Geometry check sheet. Reference: the model listing, model coordinates, mm. A direction names the side the tool comes from. Round coordinates to 2 decimals unless told otherwise and drop trailing zeros. Order: outer loops, then holes, each group sorted by start corner. A loop starts at its lowest first (then second) coordinate and runs counter-clockwise, first axis right, second up.
(1) Release check for a two-part mould opening along X. For faces 6 (the face through (17.605, 12.325, -7.465)), 7 (the face through (40, 11, 25)), 8 (the face through (49, 25, 20)) record: +X half, -X half, draft (parallel to the pull), parting line (faces both ways), or undercut.
(2) Material ranges on line 1 along Z through (x, y) = (50, 10.5); line 2 along Y through (x, z) = (42.5, 27); line 3 along Z through (x, y) = (43, 19.25), recorded low to high.
(3) Go/stop test with flat-tipped pins: pin 1 (3 mm diameter, centred on y = 22, z = 41, fed in from -X); pin 2 (1.5 mm diameter, centred on y = 9.5, z = 43, fed in from +X); pin 3 (2.5 mm diameter, centred on y = 16.5, z = -2, fed in from +X). Record where each tip stops, or that it passes through.
(4) Sectioned sample at B-B (x = 89). Record the boundary of the cut face in (y, z).
(5) Sectioned sample at A-A (y = 16). Record the boundary of the cut face in (x, z).
(6) Set-up check for faces 1 (the face through (50, 23, 25)), 2 (the face through (0, 12, 20)), 3 (the face through (82.605, 12.325, -7.535)), 4 (the face through (4.51, 12.32, 45.72)), 5 (the face through (25, 12, -2)): record each of +Z, -Z, +X, -X, +Y, -Y from which the full face is reachable in a straight line by a thin tool's end or side.
(7) Sectioned sample at D-D (x = 50). Record the boundary of the cut face in (y, z).
(8) Sectioned sample at C-C (z = 25). Record the boundary of the cut face in (x, y), plus the area to 3 significant figures.
Autodesk Fusion 360 part; units mm, degrees
sketch "Sketch1" plane through (0, 0, 0) normal (0, 1, 0) x (1, 0, 0)
  line L0 (5, 0) -> (95, 0)
  line L1 (100, -5) -> (100, -35)
  line L2 (85, -50) -> (15, -50)
  line L3 (0, -35) -> (0, -5)
  arc A0 (0, -35) -> (15, -50) centre (15, -35) ccw
  arc A1 (85, -50) -> (100, -35) centre (85, -35) ccw
  arc A2 (5, 0) -> (0, -5) centre (5, -5) ccw
  arc A3 (100, -5) -> (95, 0) centre (95, -5) ccw
  point P0 (100, 0)
  point P1 (0, -50)
  dimension "d1" = 100
  dimension "d2" = 50
  dimension "d3" = 15
  dimension "d4" = 5
extrude "Extrude1" add sketch "Sketch1" along normal blind 25
shell "Shell1" thickness 3 removed faces 1 at (61.6667, 8.3333, 50)
sketch "Sketch2" plane through (0, 0, 0) normal (0, -1, 0) x (1, 0, 0)
  arc A0 (100, 35) -> (85, 50) centre (85, 35) ccw
  line L0 (85, 50) -> (15, 50)
  arc A1 (15, 50) -> (0, 35) centre (15, 35) ccw
  line L1 (0, 35) -> (0, 5)
  arc A2 (0, 5) -> (5, 0) centre (5, 5) ccw
  line L2 (5, 0) -> (95, 0)
  arc A3 (95, 0) -> (100, 5) centre (95, 5) ccw
  line L3 (100, 5) -> (100, 35)
  line L4 (25, 0) -> (25, -5)
  line L5 (25, -5) -> (10, -10)
  line L6 (10, -10) -> (90, -10)
  line L7 (90, -10) -> (75, -5)
  line L8 (75, -5) -> (75, 0)
  circle A4 centre (50, 25) radius 10
  dimension "d8" = 5
  dimension "d9" = 5
  dimension "d10" = 50
  dimension "d11" = 80
  dimension "d12" = 10
  dimension "d13" = 20
  dimension "d14" = 50
  dimension "d15" = 25
extrude "Extrude2" cut sketch "Sketch2" against normal blind 23 contours A4
extrude "Extrude3" add sketch "Sketch2" against normal blind 25 contours L2 L4 L5 L6 L7 L8
Answer below:
1. face 6: -X half
1. face 7: undercut
1. face 8: draft
2. line 1: z = -10 to 15, 35 to 50
2. line 2: y = 23 to 25
2. line 3: z = -10 to 17.86, 32.14 to 50
3. pin 1: stops at x = 0.69
3. pin 2: stops at x = 98.13
3. pin 3: stops at x = 75
4. outline: (0, -10) - (25, -10) - (25, -9.67) - (0, -9.67) - close; (0, 0) - (25, 0) - (25, 49.46) - (0, 49.46) - close
5. outline: (0, 5) arc R5 ccw to (5, 0) - (25, 0) - (25, -5) - (10, -10) - (90, -10) - (75, -5) - (75, 0) - (95, 0) arc R5 ccw to (100, 5) - (100, 35) arc R15 ccw to (85, 50) - (15, 50) arc R15 ccw to (0, 35) - close; hole circle Ø20 at (50, 25)
6. face 1: -Y
6. face 2: +Z, -Z, -X, +Y, -Y
6. face 3: +X, +Y, -Y
6. face 4: +Z, -X, +Y, -Y
6. face 5: -X, +Y, -Y
7. outline: (0, -10) - (25, -10) - (25, 50) - (0, 50) - (0, 35) - (23, 35) - (23, 15) - (0, 15) - close
8. outline: (0, 0) - (40, 0) - (40, 23) - (60, 23) - (60, 0) - (100, 0) - (100, 25) - (0, 25) - close
8. area: 2,040 mm2
